Model file for the job. Use its own axes, mm. Face numbers are marked on the shaded views. A direction names the side the tool comes from. Coordinates: 2 decimals unless noted, no trailing zeros. Order: outer loops, then holes, each group sorted by start corner. A loop starts at its lowest first (then second) coordinate and runs counter-clockwise, first axis right, second up. Notation, with made-up numbers: M 33,43.25 L 51,43.25 A20 ccw 51,47.25 Z; hole C 65.25,-39.5 d3. An arc over 180 degrees is marked long. Return JSON: item names as keys, results as strings.
```python
from build123d import *

# Parameters (mm, degrees)
BOSS_EXTRU_1_DEPTH      = 250
ESQUISSE2_W             = 674.796104683
ESQUISSE2_H             = 230
ENL_V_MAT_EXTRU_1_DEPTH = 240
ESQUISSE3_W             = 230
ESQUISSE3_H             = 230
ENL_V_MAT_EXTRU_2_DEPTH = 40
ENL_V_MAT_EXTRU_2_DRAFT = -66
ENL_V_START             = -10
ENL_V_MAT_EXTRU_6_DEPTH = 230
ESQUISSE7_W             = 230
ESQUISSE7_H             = 230
ENL_V_MAT_EXTRU_7_DEPTH = 20
ENL_V_MAT_EXTRU_7_DRAFT = -20


with BuildPart() as part:
    # Esquisse1 → Boss.-Extru.1 (new body)
    with BuildSketch(Plane.XY):
        with BuildLine():
            add(Edge.make_bspline(
                [(0, 0.133886157), (0.167402546, 0.066889297), (0.334804949, 0)],
                knots=[1.771746973, 1.771746973, 1.771746973, 1.773247838, 1.773247838, 1.773247838], degree=2, weights=[0.999377636, 0.999688554, 1]))
            Line((0.334804949, 0), (694.461299734, 0))
            ThreePointArc((694.461299734, 0), (733.73309131, 16.26690869), (750, 55.538700266))
            Line((750, 55.538700266), (750, 194.461299734))
            ThreePointArc((750, 194.461299734), (733.73309131, 233.73309131), (694.461299734, 250))
            Line((694.461299734, 250), (0, 250))
            Line((0, 250), (0, 249.866113843))
            add(Edge.make_bspline(
                [(0, 249.866113843), (-0.167402546, 249.933110703), (-0.334804949, 250)],
                knots=[4.913528271, 4.913528271, 4.913528271, 4.914840492, 4.914840492, 4.914840492], degree=2, weights=[1, 0.999999785, 1]))
            Line((-0.334804949, 250), (-250, 250))
            add(Edge.make_bspline(
                [(-250, 250), (-312.416343553, 125.167312895), (0, 0.133886157)],
                knots=[0, 0, 0, 1.771746973, 1.771746973, 1.771746973], degree=2, weights=[1, 0.632343338, 0.999377636]))
        make_face()
    extrude(amount=BOSS_EXTRU_1_DEPTH)

    # Esquisse2 → Enlèv. mat.-Extru.1 (cut)
    with BuildSketch(Plane(origin=(0, 250, 0), x_dir=(1, 0, 0), z_dir=(0, 1, 0))):
        with Locations((347.063247392, -125)):
            Rectangle(ESQUISSE2_W, ESQUISSE2_H)
    extrude(amount=-ENL_V_MAT_EXTRU_1_DEPTH, mode=Mode.SUBTRACT)


with BuildPart() as enl_v_mat_extru_2_tool:
    # Esquisse3 → Enlèv. mat.-Extru.2 (with draft: the straight prism first)
    with BuildSketch(Plane.ZY.offset(-684.461299734)):
        with Locations((125, 125)):
            Rectangle(ESQUISSE3_W, ESQUISSE3_H)
    extrude(amount=-ENL_V_MAT_EXTRU_2_DEPTH)
    # Enlèv. mat.-Extru.2: the draft: its side faces are tilted about the plane it starts from
    enl_v_mat_extru_2_sides = [enl_v_mat_extru_2_tool.faces().sort_by_distance(p)[0] for p in [
        (704.461299734, 125, 10),
        (704.461299734, 10, 125),
        (704.461299734, 125, 240),
        (704.461299734, 240, 125),
    ]]
    draft(enl_v_mat_extru_2_sides, Plane.ZY.offset(-684.461299734), ENL_V_MAT_EXTRU_2_DRAFT)


with BuildPart() as part_1:
    add(part.part)

    # Enlèv. mat.-Extru.2: cut by enl_v_mat_extru_2_tool
    add(enl_v_mat_extru_2_tool.part, mode=Mode.SUBTRACT)

    # Esquisse5 → Enlèv. mat.-Extru.6 (cut)
    with BuildSketch(Plane.XY.offset(250).offset(ENL_V_START)):
        with BuildLine():
            Line((0.013392186, 240.000008968), (0.321682976, 9.798221826))
            add(Edge.make_bspline(
                [(-243.578112703, 240.000000104), (-281.360738576, 124.899105152), (0.321682976, 9.798221826)],
                knots=[0.057124258, 0.057124258, 0.057124258, 1.763084739, 1.763084739, 1.763084739], degree=2, weights=[1, 0.657741222, 1]))
            Line((-243.578112703, 240.000000104), (0.013392186, 240.000008968))
        make_face()
    extrude(amount=-ENL_V_MAT_EXTRU_6_DEPTH, mode=Mode.SUBTRACT)


with BuildPart() as enl_v_mat_extru_7_tool:
    # Esquisse7 → Enlèv. mat.-Extru.7 (with draft: the straight prism first)
    with BuildSketch(Plane(origin=(9.665195051, 0, 0), x_dir=(0, 0, -1), z_dir=(1, 0, 0))):
        with Locations((-125, 125)):
            Rectangle(ESQUISSE7_W, ESQUISSE7_H)
    extrude(amount=-ENL_V_MAT_EXTRU_7_DEPTH)
    # Enlèv. mat.-Extru.7: the draft: its side faces are tilted about the plane it starts from
    enl_v_mat_extru_7_sides = [enl_v_mat_extru_7_tool.faces().sort_by_distance(p)[0] for p in [
        (-0.334804949, 125, 10),
        (-0.334804949, 240, 125),
        (-0.334804949, 125, 240),
        (-0.334804949, 10, 125),
    ]]
    draft(enl_v_mat_extru_7_sides, Plane(origin=(9.665195051, 0, 0), x_dir=(0, 0, -1), z_dir=(1, 0, 0)), ENL_V_MAT_EXTRU_7_DRAFT)


with BuildPart() as part_2:
    add(part_1.part)

    # Enlèv. mat.-Extru.7: cut by enl_v_mat_extru_7_tool
    add(enl_v_mat_extru_7_tool.part, mode=Mode.SUBTRACT)


solid = part_2.part
```
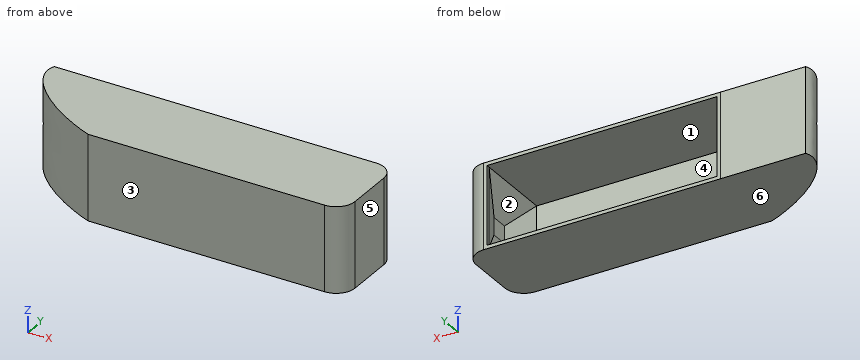
Item 1: Wall check: line 1 (Z direction, x = 247, y = 156); line 2 (Y direction, x = 89, z = 116.5); line 3 (X direction, y = 193, z = 205). Give the ranges that are in metal, low to high.
Check result:
{"line 1": "z = 0 to 10, 240 to 250", "line 2": "y = 0 to 10", "line 3": "x = -247.19 to -237.75, 700.04 to 750"}
Item 2: 3-axis set-ups, long thin cutter, end or side, ignore diameter. For the marked faces 1, 2 and 3: which of +Z, -Z, +X, -X, +Y, -Y reach the whole face in a straight line?
Check result:
{"face 1": "+Y", "face 2": "none", "face 3": "+Z, -Z, +X, -X, -Y"}
Item 3: Pull direction Z, two halves, no side cores. Call the marked faces 4, 5 and 6: +Z half, -Z half, draft (parallel to the pull), parting line (faces both ways), or undercut.
Check result:
{"face 4": "undercut", "face 5": "draft", "face 6": "-Z half"}
Item 4: Saw through at A-A (x = 49.5). Write the cut outline in (y, z).
Check result:
{"outline": "M 0,0 L 250,0 L 250,10 L 10,10 L 10,240 L 250,240 L 250,250 L 0,250 Z"}
Item 5: Drop flat-ended pins along their axis: pin 1 Ø8 at (y, z) = (247.5, 104) entering from +X; pin 2 Ø25 at (y, z) = (134, 128) entering from -X; pin 3 Ø10 at (y, z) = (175, 107) entering from -X. Give the stop position or say it passes through.
Check result:
{"pin 1": "stops at x = 720.53", "pin 2": "stops at x = -217.28", "pin 3": "stops at x = -240.75"}
